Geometry: final body of the model. Coordinates: model frame, mm. A direction names the side the tool comes from. Give positions to 0.01 mm unless a question says otherwise; leave off trailing zeros. Order: outer loops, then holes, each group sorted by start corner. A loop starts at its lowest first (then second) coordinate and runs counter-clockwise, first axis right, second up. Notation, with made-up numbers: (87.5, 36) -> (102.5, 36) arc R34 ccw to (102.5, 68) -> close; hole circle Ø3 at (-30.5, 45). An arc over 180 degrees is marked (long way). Write item = value, one per line.
```python
from build123d import *

# Parameters (mm, degrees)
FILLET1_R           = 0.5
SKETCH5_R           = 5.5
CUT_EXTRUDE1_DEPTH  = 1
FILLET2_R           = 0.5
CUT_EXTRUDE2_START  = -1
SKETCH6_R           = 5.5
CUT_EXTRUDE2_DEPTH  = 1
FILLET3_R           = 0.5
SKETCH8_R           = 4.3
SKETCH8_R_2         = 4
BOSS_EXTRUDE4_DEPTH = 0.3
BOSS_EXTRUDE5_START = 0.3
SKETCH9_R           = 4.3
SKETCH9_R_2         = 4
BOSS_EXTRUDE5_DEPTH = 0.3


with BuildPart() as part:
    # Sketch4 → Revolve1 (revolve)
    with BuildSketch(Plane(origin=(0, 0, 0), x_dir=(0, 0, -1), z_dir=(1, 0, 0)), mode=Mode.PRIVATE) as revolve1_sk:
        Polygon((-0.139006256, 4), (23.860993744, 4), (23.860993744, 7), (20.610993744, 7), (20.610993744, 6.291984931), (19.510993744, 6.291984931), (19.510993744, 7), (4.210993744, 7), (4.210993744, 6.386905477), (3.110993744, 6.386905477), (3.110993744, 7), (-0.139006256, 7), align=None)
    revolve(revolve1_sk.sketch.rotate(Axis((0, 0, 0), (0, 0, -1)), 90), axis=Axis((0, 0, 0), (0, 0, -1)))

    # Fillet1
    fillet1_edges = [part.edges().sort_by_distance(p)[0] for p in [
        (-7, 0, -23.860993744),
        (-7, 0, 0.139006256),
    ]]
    fillet(fillet1_edges, radius=FILLET1_R)

    # Sketch5 → Cut-Extrude1 (cut)
    with BuildSketch(Plane.XY.offset(0.139006256)):
        Circle(SKETCH5_R)
    extrude(amount=-CUT_EXTRUDE1_DEPTH, mode=Mode.SUBTRACT)

    # Fillet2
    fillet2_edges = [part.edges().sort_by_distance(p)[0] for p in [
        (-5.5, 0, 0.139006256),
    ]]
    fillet(fillet2_edges, radius=FILLET2_R)

    # Sketch6 → Cut-Extrude2 (cut)
    with BuildSketch(Plane(origin=(0, 0, -23.860993744), x_dir=(-1, 0, 0), z_dir=(0, 0, -1)).offset(CUT_EXTRUDE2_START)):
        with Locations(Location((0, 0, 0), (0, 0, 180))):
            Circle(SKETCH6_R)
    extrude(amount=CUT_EXTRUDE2_DEPTH, mode=Mode.SUBTRACT)

    # Fillet3
    fillet3_edges = [part.edges().sort_by_distance(p)[0] for p in [
        (-5.5, 0, -23.860993744),
    ]]
    fillet(fillet3_edges, radius=FILLET3_R)

    # Sketch8 → Boss-Extrude4 (add)
    with BuildSketch(Plane.XY.offset(-0.860993744)):
        Circle(SKETCH8_R)
        Circle(SKETCH8_R_2, mode=Mode.SUBTRACT)
    extrude(amount=BOSS_EXTRUDE4_DEPTH)

    # Sketch9 → Boss-Extrude5 (add)
    with BuildSketch(Plane(origin=(0, 0, -22.860993744), x_dir=(-1, 0, 0), z_dir=(0, 0, -1)).offset(BOSS_EXTRUDE5_START)):
        with Locations(Location((0, 0, 0), (0, 0, 180))):
            Circle(SKETCH9_R)
        with Locations(Location((0, 0, 0), (0, 0, 180))):
            Circle(SKETCH9_R_2, mode=Mode.SUBTRACT)
    extrude(amount=-BOSS_EXTRUDE5_DEPTH)


solid = part.part
```
1) Reachability of faces 5 (the face through (2, 6, 0.139)), 6 (the face through (-1.19, -5.37, -0.61)), 7 (the face through (3.23, 6.21, -11.75)), 8 (the face through (-6, -3, -20.611)), 9 (the face through (2, 4, -22.861)) from +Z, -Z, +X, -X, +Y, -Y: full face, straight path, thin tool, end or side. Return the list, or none.
Check sheet entries:
face_5 = +Z, +X, -X, +Y, -Y
face_6 = +Z
face_7 = +Z, -Z
face_8 = none
face_9 = -Z
2) Mould query, pull axis Z, two halves, no side actions, for faces 1 (the face through (6, -3, -19.511)), 2 (the face through (-1.19, 5.37, -23.11)), 3 (the face through (3, 6, -4.211)), 4 (the face through (-2, 6, -23.861)). Classes: +Z half, -Z half, draft (parallel to the pull), parting line (faces both ways), or undercut.
Check sheet entries:
face_1 = undercut
face_2 = draft
face_3 = undercut
face_4 = -Z half
3) First-contact query: P1, Ø1, axis at y = 2, z = -16, coming from the +X side; P2, Ø3, axis at x = 3, y = -3, coming from the -Z side; P3, Ø6, axis at y = 3.5, z = -21, coming from the +X side; P4, Ø3.5, axis at x = -2, y = 0.5, coming from the +Z side. Flat tips, straight axial feed; report the tip coordinate or a pass-through.
Check sheet entries:
P1 = 6.84
P2 = -23.79
P3 = 6.98
P4 = through
4) Line query: line 1 (Y direction, x = 0, z = -0.65); line 2 (Y direction, x = 0, z = -13.25); line 3 (Z direction, x = -5, y = -1.75). Output: solid intervals per line, ascending. Write a range as from..to.
Check sheet entries:
line_1 = -7..-5.5, -4.3..-4, 4..4.3, 5.5..7
line_2 = -7..-4, 4..7
line_3 = -22.86..-0.86
5) Section query A-A (z = -5.75). Output: boundary loops of the cut face in (x, y), plus the area to 3 significant figures.
Check sheet entries:
outline = circle Ø14 at (0, 0); hole circle Ø8 at (0, 0)
area = 104 mm²
